Verification items for the finished model (mm, model axes). Face numbers are marked on the shaded views. A direction names the side the tool comes from. Coordinates: 2 decimals unless noted, no trailing zeros. Order: outer loops, then holes, each group sorted by start corner. A loop starts at its lowest first (then second) coordinate and runs counter-clockwise, first axis right, second up. Notation, with made-up numbers: M -31,-0.75 L 7,-0.75 A11 ccw 7,5.25 Z; hole C -36.5,68 d10. An arc over 180 degrees is marked long. Answer as a JSON object with one key per item and string values. Group by question number.
(1) Access from +Z, -Z, +X, -X, +Y, -Y to the whole of each face (thin tool, end or side, straight path). Record for the marked faces 4, 5, 6 and 7.
(2) Cross-section at D-D (z = -1). Enter the section's corners in (x, y), plus the area to 3 significant figures.
(3) Cross-section at A-A (y = -12.75). Count the separate pieces of the cut face and the enclosed holes in it, plus the area to 3 significant figures.
(4) Cross-section at C-C (z = -39). Enter the section's corners in (x, y), plus the area to 3 significant figures.
(5) Cross-section at B-B (x = -3). Enter the section's corners in (y, z).
(6) Material ranges on line 1 (X direction, y = -1, z = -19); line 2 (X direction, y = -45.25, z = 26); line 3 (Y direction, x = 24, z = -10.5), recorded low to high.
(7) Mould release check, pull along X, two halves, no side actions. Record for the marked faces 1, 2 and 3: released by +X, released by -X, zero draft, split by the parting line, or undercut.
(8) Gauge pin test, flat ends, axial feed: pin 1 Ø8 at (x, y) = (-16.5, -37.5) entering from +Z; pin 2 Ø6.5 at (x, y) = (16.25, -12.75) entering from -Z; pin 3 Ø12 at (y, z) = (-47.5, -33) entering from -X; pin 4 Ø10 at (x, z) = (17, -28.5) entering from +Y. Record the tip position at first contact, or that the pin passes through.
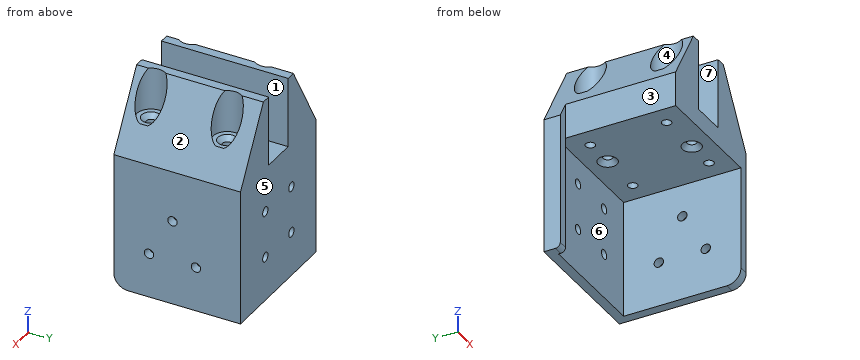
from build123d import *

# Parameters (mm, degrees)
PAD006_DEPTH    = 54
SKETCH035_W     = 50
SKETCH035_H     = 50
POCKET015_DEPTH = 50
SKETCH036_W     = 47
SKETCH036_H     = 50
POCKET016_DEPTH = 50
FILLET008_R     = 6
FILLET009_R     = 2
SKETCH037_W     = 4
SKETCH037_H     = 47
POCKET017_DEPTH = 25
SKETCH038_R     = 2
POCKET018_DEPTH = 50
CHAMFER008_SIZE = 2
SKETCH039_R     = 6
POCKET019_DEPTH = 50
CHAMFER009_SIZE = 2
SKETCH040_R     = 2
POCKET020_DEPTH = 50
SKETCH041_R     = 2
POCKET021_DEPTH = 10


with BuildPart() as part:
    # Sketch034 → Pad006 (new body)
    with BuildSketch(Plane.XZ):
        Polygon((-7.5, 0), (7.5, 0), (7.5, 30), (11.5, 30), (29, 0), (29, -58), (-29, -58), (-29, 0), (-11.5, 30), (-7.5, 30), align=None)
    extrude(amount=PAD006_DEPTH)

    # Sketch035 → Pocket015 (cut)
    with BuildSketch(Plane.XZ.offset(4)):
        with Locations((0, -33)):
            Rectangle(SKETCH035_W, SKETCH035_H)
    extrude(amount=POCKET015_DEPTH, mode=Mode.SUBTRACT)

    # Sketch036 → Pocket016 (cut)
    with BuildSketch(Plane.YZ):
        with Locations((-30.5, -33)):
            Rectangle(SKETCH036_W, SKETCH036_H)
    extrude(amount=-POCKET016_DEPTH, mode=Mode.SUBTRACT)

    # Fillet008
    fillet008_edges = [part.edges().sort_by_distance(p)[0] for p in [
        (27, -54, -58),
    ]]
    fillet(fillet008_edges, radius=FILLET008_R)

    # Fillet009
    fillet009_edges = [part.edges().sort_by_distance(p)[0] for p in [
        (-27, -7, -58),
    ]]
    fillet(fillet009_edges, radius=FILLET009_R)

    # Sketch037 → Pocket017 (cut, symmetric)
    with BuildSketch(Plane.XY):
        with Locations((-27, -30.5)):
            Rectangle(SKETCH037_W, SKETCH037_H)
    extrude(amount=POCKET017_DEPTH, both=True, mode=Mode.SUBTRACT)

    # Sketch038 → Pocket018 (cut, symmetric)
    with BuildSketch(Plane.XY):
        with Locations((-16.25, -12.75)):
            Circle(SKETCH038_R)
        with Locations((-16.25, -45.25)):
            Circle(SKETCH038_R)
        with Locations((16.25, -45.25)):
            Circle(SKETCH038_R)
        with Locations((16.25, -12.75)):
            Circle(SKETCH038_R)
        with Locations((-3, -12.75)):
            Circle(SKETCH038_R)
        with Locations((3, -45.25)):
            Circle(SKETCH038_R)
    extrude(amount=POCKET018_DEPTH, both=True, mode=Mode.SUBTRACT)

    # Chamfer008
    chamfer008_edges = [part.edges().sort_by_distance(p)[0] for p in [
        (1, -45.25, -8),
        (-5, -12.75, -8),
    ]]
    chamfer(chamfer008_edges, length=CHAMFER008_SIZE)

    # Sketch039 → Pocket019 (cut)
    with BuildSketch(Plane.XY.offset(12)):
        with Locations((-16.25, -12.75)):
            Circle(SKETCH039_R)
        with Locations((-16.25, -45.25)):
            Circle(SKETCH039_R)
        with Locations((16.25, -45.25)):
            Circle(SKETCH039_R)
        with Locations((16.25, -12.75)):
            Circle(SKETCH039_R)
    extrude(amount=POCKET019_DEPTH, mode=Mode.SUBTRACT)

    # Chamfer009
    chamfer009_edges = [part.edges().sort_by_distance(p)[0] for p in [
        (-18.25, -45.25, 12),
        (-18.25, -12.75, 12),
        (14.25, -45.25, 12),
        (14.25, -12.75, 12),
    ]]
    chamfer(chamfer009_edges, length=CHAMFER009_SIZE)

    # Sketch040 → Pocket020 (cut)
    with BuildSketch(Plane.YZ):
        with Locations((-29, -21.679492)):
            Circle(SKETCH040_R)
        with Locations((-39, -39)):
            Circle(SKETCH040_R)
        with Locations((-19, -39)):
            Circle(SKETCH040_R)
    extrude(amount=POCKET020_DEPTH, mode=Mode.SUBTRACT)

    # Sketch041 → Pocket021 (cut)
    with BuildSketch(Plane.XZ):
        with Locations((-10, -19)):
            Circle(SKETCH041_R)
        with Locations((10, -19)):
            Circle(SKETCH041_R)
        with Locations((-10, -39)):
            Circle(SKETCH041_R)
        with Locations((10, -39)):
            Circle(SKETCH041_R)
    extrude(amount=POCKET021_DEPTH, mode=Mode.SUBTRACT)


solid = part.part
Taken from the geometry:
{
 "1": {"face 4": "+Z", "face 5": "+Z, -Z, +X, -X, +Y", "face 6": "-Z, -Y", "face 7": "+Z, +Y, -Y"},
 "2": {"outline": "M -29,-7 L -25,-7 L -25,-54 L 29,-54 L 29,0 L -29,0 Z; hole C -16.25,-45.25 d4; hole C -16.25,-12.75 d4; hole C -3,-12.75 d4; hole C 3,-45.25 d4; hole C 16.25,-45.25 d4; hole C 16.25,-12.75 d4", "area": "2,870 mm²"},
 "3": {"separate pieces": "4", "enclosed holes": "0", "area": "945 mm²"},
 "4": {"outline": "M -29,-7 L -25,-7 L -25,-4 L -12,-4 L -12,0 L -29,0 Z; M -8,-4 L 8,-4 L 8,0 L -8,0 Z; M 12,-4 L 25,-4 L 25,-17 L 29,-17 L 29,0 L 12,0 Z; M 25,-54 L 29,-54 L 29,-41 L 25,-41 Z; M 25,-37 L 29,-37 L 29,-21 L 25,-21 Z", "area": "380 mm²"},
 "5": {"outline": "M -54,-8 L -16.75,-8 L -14.75,-6 L -14.75,0 L -54,0 Z; M -10.75,-6 L -8.75,-8 L -4,-8 L -4,-58 L 0,-58 L 0,0 L -10.75,0 Z"},
 "6": {"line 1": "x = -29 to -12, -8 to 8, 12 to 29", "line 2": "x = -10.25 to -7.5, 7.5 to 10.25", "line 3": "y = -4 to 0"},
 "7": {"face 1": "undercut", "face 2": "released by +X", "face 3": "released by -X"},
 "8": {"pin 1": "stops at z = 28.29", "pin 2": "stops at z = -8", "pin 3": "stops at x = 25", "pin 4": "stops at y = 0"}
}
